Can you work these out from the model? Positions are in its coordinate system, mm. A direction names the side the tool comes from. Give positions to 0.01 mm unless a question says otherwise; leave off trailing zeros. Write each loop counter-clockwise with the first axis right and the second up, starting at its lowest first coordinate (ties: lowest second). Pieces come first, ordered by that corner, then holes.
from build123d import *

# Parameters (mm, degrees)
SKETCH_W             = 40
SKETCH_H             = 20
PAD_DEPTH            = 10
POCKET_DEPTH         = 40.001
SKETCH002_W          = 10
SKETCH002_H          = 6
POCKET001_DEPTH      = 8.001
SKETCH003_R          = 2
POCKET002_DEPTH      = 3
POCKET002_DEPTH_BACK = -13
SKETCH004_W          = 16
SKETCH004_H          = 4
POCKET003_DEPTH      = 3
CHAMFER_SIZE         = 1
CHAMFER001_SIZE      = 1
CHAMFER002_SIZE      = 1
CHAMFER003_SIZE      = 1
CHAMFER004_SIZE      = 1
CHAMFER005_SIZE      = 1
CHAMFER006_SIZE      = 1
SKETCH005_W          = 16
SKETCH005_H          = 12
POCKET004_DEPTH      = 5


with BuildPart() as part:
    # Sketch → Pad (new body)
    with BuildSketch(Plane.XY):
        with Locations((20, 10)):
            Rectangle(SKETCH_W, SKETCH_H)
    extrude(amount=PAD_DEPTH)

    # Sketch001 (on Face2 of Pad) → Pocket (cut, through all)
    with BuildSketch(Plane.YZ.offset(40)):
        with BuildLine():
            Line((0, 8), (4, 8))
            Line((4, 8), (4, 5))
            ThreePointArc((4, 5), (6, 3), (8, 5))
            Line((8, 8), (8, 5))
            Line((8, 8), (25, 8))
            Line((25, 8), (25, 10))
            Line((25, 10), (0, 10))
            Line((0, 10), (0, 8))
        make_face()
    extrude(amount=-POCKET_DEPTH, mode=Mode.SUBTRACT)

    # Sketch002 (on Face4 of Pocket) → Pocket001 (cut, through all)
    with BuildSketch(Plane.XY.offset(8)):
        with Locations((30, 17)):
            Rectangle(SKETCH002_W, SKETCH002_H)
    extrude(amount=-POCKET001_DEPTH, mode=Mode.SUBTRACT)

    # Sketch003 (on Face9 of Pocket001) → Pocket002 (cut, two sides)
    with BuildSketch(Plane(origin=(35, 0, 0), x_dir=(0, -1, 0), z_dir=(-1, 0, 0))) as pocket002_sk:
        with Locations((-17, 5)):
            Circle(SKETCH003_R)
    extrude(amount=-POCKET002_DEPTH, mode=Mode.SUBTRACT)
    extrude(pocket002_sk.sketch, amount=-POCKET002_DEPTH_BACK, mode=Mode.SUBTRACT)

    # Sketch004 (on Face1 of Pocket002) → Pocket003 (cut)
    with BuildSketch(Plane(origin=(0, 20, 0), x_dir=(-1, 0, 0), z_dir=(0, 1, 0))):
        with Locations((-30, 5)):
            Rectangle(SKETCH004_W, SKETCH004_H)
    extrude(amount=-POCKET003_DEPTH, mode=Mode.SUBTRACT)

    # Chamfer
    chamfer_edges = [part.edges().sort_by_distance(p)[0] for p in [
        (20, 0, 8),
    ]]
    chamfer(chamfer_edges, length=CHAMFER_SIZE)

    # Chamfer001
    chamfer001_edges = [part.edges().sort_by_distance(p)[0] for p in [
        (12.5, 20, 8),
    ]]
    chamfer(chamfer001_edges, length=CHAMFER001_SIZE)

    # Chamfer002
    chamfer002_edges = [part.edges().sort_by_distance(p)[0] for p in [
        (37.5, 20, 8),
    ]]
    chamfer(chamfer002_edges, length=CHAMFER002_SIZE)

    # Chamfer003
    chamfer003_edges = [part.edges().sort_by_distance(p)[0] for p in [
        (0, 13.5, 8),
    ]]
    chamfer(chamfer003_edges, length=CHAMFER003_SIZE)

    # Chamfer004
    chamfer004_edges = [part.edges().sort_by_distance(p)[0] for p in [
        (0, 2.5, 8),
    ]]
    chamfer(chamfer004_edges, length=CHAMFER004_SIZE)

    # Chamfer005
    chamfer005_edges = [part.edges().sort_by_distance(p)[0] for p in [
        (20.5, 8, 8),
    ]]
    chamfer(chamfer005_edges, length=CHAMFER005_SIZE)

    # Chamfer006
    chamfer006_edges = [part.edges().sort_by_distance(p)[0] for p in [
        (20.5, 4, 8),
    ]]
    chamfer(chamfer006_edges, length=CHAMFER006_SIZE)

    # Sketch005 (on Face11 of Chamfer006) → Pocket004 (cut)
    with BuildSketch(Plane(origin=(0, 0, 0), x_dir=(1, 0, 0), z_dir=(0, 0, -1))):
        with Locations((12, -10)):
            Rectangle(SKETCH005_W, SKETCH005_H)
    extrude(amount=-POCKET004_DEPTH, mode=Mode.SUBTRACT)


solid = part.part
(1) Will these pins go through, and if not, where does the flat tip stop? P1, Ø3.5, axis at x = 24, y = 18, coming from the -Z side; P2, Ø4, axis at x = 16, y = 10.5, coming from the -Z side; P3, Ø2, axis at x = 31, z = 1, coming from the +Y side.
Returned:
P1: stops at z = 0
P2: stops at z = 5
P3: stops at y = 14
(2) Imagine slicing it at A-A, the plane y = 6. Write out the boundary of the cut face in (x, z), plus the area to 3 significant figures.
Returned:
outline: (0, 0) - (4, 0) - (4, 3) - (0, 3) - close; (20, 0) - (40, 0) - (40, 3) - (20, 3) - close
area: 72.0 mm2
(3) Imagine slicing it at C-C, the plane z = 1. Write out the boundary of the cut face in (x, y).
Returned:
outline: (0, 0) - (40, 0) - (40, 20) - (35, 20) - (35, 14) - (25, 14) - (25, 20) - (0, 20) - close; hole (4, 4) - (20, 4) - (20, 16) - (4, 16) - close
(4) Imagine slicing it at B-B, the plane x = 13.5. Write out the boundary of the cut face in (y, z), plus the area to 3 significant figures.
Returned:
outline: (0, 0) - (4, 0) - (4, 7) - (3, 8) - (1, 8) - (0, 7) - close; (8, 5) - (16, 5) - (16, 0) - (20, 0) - (20, 7) - (19, 8) - (9, 8) - (8, 7) - close
area: 86.0 mm2
(5) Imagine slicing it at D-D, the plane z = 7.5. Write out the boundary of the cut face in (x, y), plus the area to 3 significant figures.
Returned:
outline: (0.5, 0.5) - (40, 0.5) - (40, 3.5) - (0.5, 3.5) - close; (0.5, 8.5) - (40, 8.5) - (40, 19.5) - (35, 19.5) - (35, 14) - (25, 14) - (25, 19.5) - (0.5, 19.5) - close
area: 498 mm2
(6) If we mould it in two halves opening along X, with no side actions, what happens to faces 6 (the face through (35, 16, 3)), 7 (the face through (0, 10, 3)), 8 (the face through (20, 8, 6))? For each: +X half, -X half, draft (parallel to the pull), parting line (faces both ways), or undercut.
Returned:
face 6: undercut
face 7: -X half
face 8: draft
(7) For faces 1 (the face through (12, 16, 2)), 2 (the face through (36, 15, 5)), 3 (the face through (16, 4, 4)), 4 (the face through (25, 16, 3)), 5 (the face through (20.3, 3.5, 7.5)), which set-ups out of +Z, -Z, +X, -X, +Y, -Y let a thin tool reach every point of the face, with its end or its side?
Returned:
face 1: -Z
face 2: +Y
face 3: +Z
face 4: +Z, -Z, +Y
face 5: +Z, +X, -X
(8) If I drill on L1, parallel to X at y = 14.5, z = 4; L2, parallel to Y at x = 16.5, z = 1.5; L3, parallel to X at y = 9.5, z = 2, over which ranges is the centre line in solid material (lowest first)?
Returned:
L1: x = 0 to 4, 20 to 25, 35 to 40
L2: y = 0 to 4, 16 to 20
L3: x = 0 to 4, 20 to 40
